Drawing for the job (mm, zero at the part's lowest x, y, z). Round coordinates to 2 decimals unless told otherwise and drop trailing zeros. Loops run counter-clockwise (first coordinate to the right, second up) from the corner with the lowest first, then second, coordinate; pieces in that order, holes last.
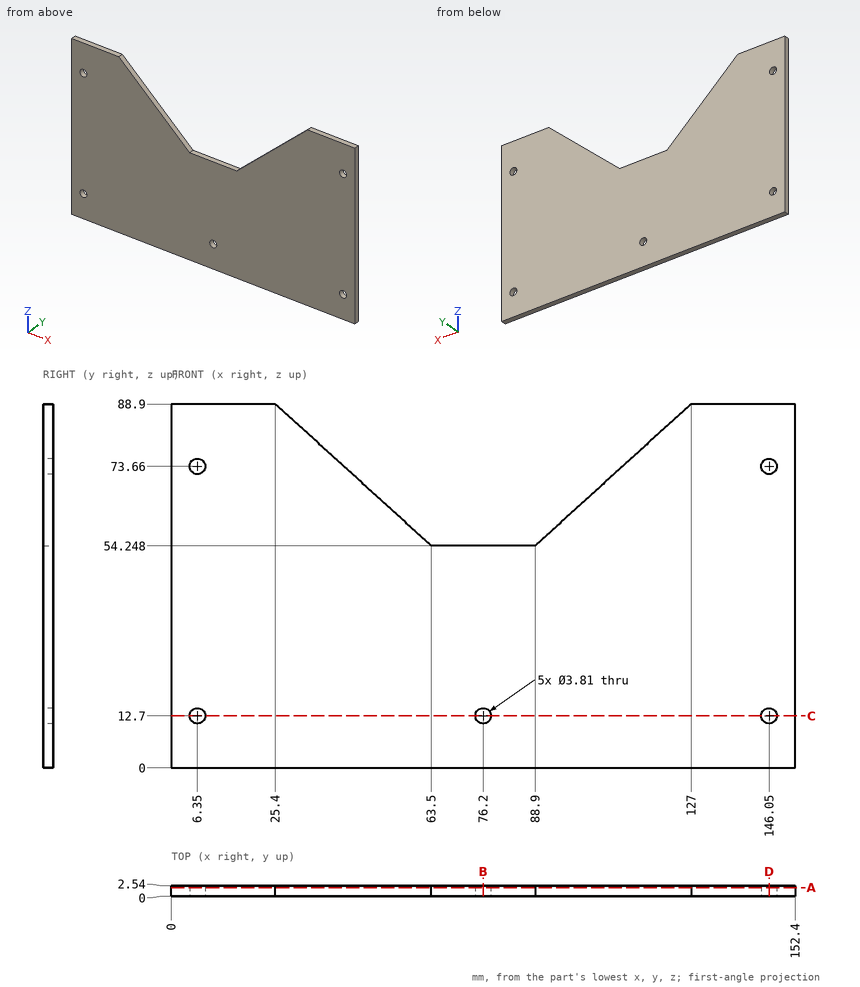
Q1. Flat gauge pins, fed straight in: P1, Ø3, axis at x = 6.35, z = 73.66, coming from the +Y side; P2, Ø1.3, axis at x = 78.5, y = 2, coming from the +Z side. Where does each tip first touch, or does it go through?
Q2. Probe line 1 (Z direction, x = 146.05, y = 0.7) (3 decimals); line 2 (X direction, y = 0.75, z = 12); line 3 (X direction, y = 1.2, z = 75). List the from-to ranges inside material, lowest first.
Q3. Slice it at D-D on x = 146.05. Give the cut face in (y, z) (3 decimals), plus the area to 3 significant figures.
Q4. Slice it at A-A on y = 2.1. Give the cut face in (x, z) (3 decimals), plus the area to 3 significant figures.
Q5. Slice it at C-C on z = 12.7. Give the cut face in (x, y) (3 decimals).
Q6. Slice it at B-B on x = 76.2. Give the cut face in (y, z) (3 decimals), plus the area to 3 significant figures.
Reply:
1. P1: passes through
1. P2: stops at z = 54.25
2. line 1: z = 0 to 10.795, 14.605 to 71.755, 75.565 to 88.9
2. line 2: x = 0 to 4.58, 8.12 to 74.43, 77.97 to 144.28, 147.82 to 152.4
2. line 3: x = 0 to 5, 7.7 to 40.68, 111.72 to 144.7, 147.4 to 152.4
3. outline: (0, 0) - (2.54, 0) - (2.54, 10.795) - (0, 10.795) - close; (0, 14.605) - (2.54, 14.605) - (2.54, 71.755) - (0, 71.755) - close; (0, 75.565) - (2.54, 75.565) - (2.54, 88.9) - (0, 88.9) - close
3. area: 206 mm2
4. outline: (0, 0) - (152.4, 0) - (152.4, 88.9) - (127, 88.9) - (88.9, 54.248) - (63.5, 54.248) - (25.4, 88.9) - (0, 88.9) - close; hole circle Ø3.81 at (6.35, 12.7); hole circle Ø3.81 at (6.35, 73.66); hole circle Ø3.81 at (76.2, 12.7); hole circle Ø3.81 at (146.05, 12.7); hole circle Ø3.81 at (146.05, 73.66)
4. area: 11,300 mm2
5. outline: (0, 0) - (4.445, 0) - (4.445, 2.54) - (0, 2.54) - close; (8.255, 0) - (74.295, 0) - (74.295, 2.54) - (8.255, 2.54) - close; (78.105, 0) - (144.145, 0) - (144.145, 2.54) - (78.105, 2.54) - close; (147.955, 0) - (152.4, 0) - (152.4, 2.54) - (147.955, 2.54) - close
6. outline: (0, 0) - (2.54, 0) - (2.54, 10.795) - (0, 10.795) - close; (0, 14.605) - (2.54, 14.605) - (2.54, 54.248) - (0, 54.248) - close
6. area: 128 mm2
